Design review of the part built by this model. Coordinates are the model's own, in mm. Coordinates: 2 decimals unless noted, no trailing zeros. Write each loop counter-clockwise with the first axis right and the second up, starting at its lowest first coordinate (ties: lowest second). Pieces come first, ordered by that corner, then holes. Notation, with made-up numbers: (-20, -26.75) - (38, -26.75) arc R25 ccw to (38, -9.75) - close; hole circle Ø1 at (2, 9.5). An arc over 180 degrees is marked (long way). One line per item, written item: value.
from build123d import *

# Parameters (mm, degrees)
BOSS_EXTRUDE1_DEPTH                  = 166.33825
F_10_32_TAPPED_HOLE1_D               = 4.0386
F_10_32_TAPPED_HOLE1_DEPTH           = 16.34744
F_10_32_TAPPED_HOLE1_TIP             = 1.213317848
F_10_32_TAPPED_HOLE1_ON_FACE_2_D     = 4.0386
F_10_32_TAPPED_HOLE1_ON_FACE_2_DEPTH = 16.34744
F_10_32_TAPPED_HOLE1_ON_FACE_2_TIP   = 1.213317848
SKETCH5_W                            = 0.889
SKETCH5_H                            = 1.0033


with BuildPart() as part:
    # Sketch1 → Boss-Extrude1 (new, symmetric)
    with BuildSketch(Plane.XY):
        with BuildLine():
            ThreePointArc((0.93173274, 6.79441227), (0, 6.858), (-0.93173274, 6.79441227))
            Line((-0.93173274, 6.79441227), (-5.41826726, 4.204110358))
            ThreePointArc((-5.41826726, 4.204110358), (-5.939202219, 3.429), (-6.35, 2.590301913))
            Line((-6.35, 2.590301913), (-6.35, -2.590301913))
            ThreePointArc((-6.35, -2.590301913), (-5.939202219, -3.429), (-5.41826726, -4.204110358))
            Line((-5.41826726, -4.204110358), (-0.93173274, -6.79441227))
            ThreePointArc((-0.93173274, -6.79441227), (0, -6.858), (0.93173274, -6.79441227))
            Line((0.93173274, -6.79441227), (5.41826726, -4.204110358))
            ThreePointArc((5.41826726, -4.204110358), (5.939202219, -3.429), (6.35, -2.590301913))
            Line((6.35, -2.590301913), (6.35, 2.590301913))
            ThreePointArc((6.35, 2.590301913), (5.939202219, 3.429), (5.41826726, 4.204110358))
            Line((5.41826726, 4.204110358), (0.93173274, 6.79441227))
        make_face()
    extrude(amount=BOSS_EXTRUDE1_DEPTH, both=True)

    # #10-32 Tapped Hole1
    with Locations(Plane.XY.offset(166.33825)):
        with Locations((0, 0)):
            Hole(F_10_32_TAPPED_HOLE1_D / 2, depth=F_10_32_TAPPED_HOLE1_DEPTH)
            with Locations((0, 0, -(F_10_32_TAPPED_HOLE1_DEPTH + F_10_32_TAPPED_HOLE1_TIP / 2))):  # 118° drill point
                Cone(0, F_10_32_TAPPED_HOLE1_D / 2, F_10_32_TAPPED_HOLE1_TIP, mode=Mode.SUBTRACT)

    # #10-32 Tapped Hole1 on face 2
    with Locations(Plane(origin=(0, 0, -166.33825), x_dir=(-1, 0, 0), z_dir=(0, 0, -1))):
        with Locations((0, 0)):
            Hole(F_10_32_TAPPED_HOLE1_ON_FACE_2_D / 2, depth=F_10_32_TAPPED_HOLE1_ON_FACE_2_DEPTH)
            with Locations((0, 0, -(F_10_32_TAPPED_HOLE1_ON_FACE_2_DEPTH + F_10_32_TAPPED_HOLE1_ON_FACE_2_TIP / 2))):  # 118° drill point
                Cone(0, F_10_32_TAPPED_HOLE1_ON_FACE_2_D / 2, F_10_32_TAPPED_HOLE1_ON_FACE_2_TIP, mode=Mode.SUBTRACT)

    # Sketch5 → Cut-Revolve1 (revolve, cut)
    with BuildSketch(Plane(origin=(0, 0, 0), x_dir=(0, 0, -1), z_dir=(1, 0, 0)), mode=Mode.PRIVATE) as cut_revolve1_sk:
        with Locations((-164.30625, 6.35635)):
            Rectangle(SKETCH5_W, SKETCH5_H)
    revolve(cut_revolve1_sk.sketch.rotate(Axis((0, 0, 165.047176272), (0, 0, -1)), 90), axis=Axis((0, 0, 165.047176272), (0, 0, -1)), mode=Mode.SUBTRACT)


solid = part.part
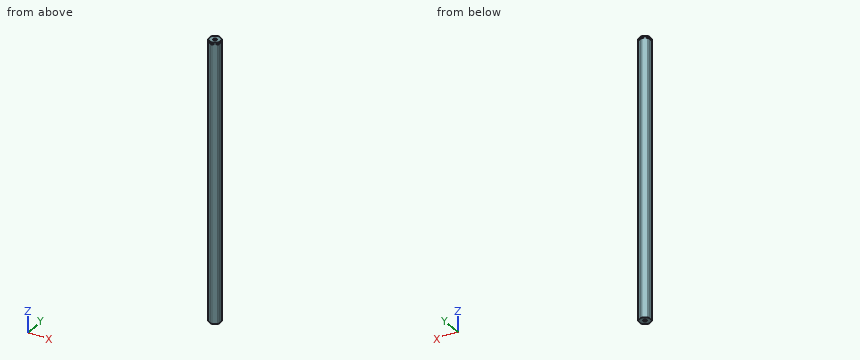
1. Insertion check: pin 1 Ø6 at (x, z) = (-4, -69) entering from +Y (3 decimals); pin 2 Ø3 at (x, z) = (-0.5, 48) entering from +Y. Each pin has a flat end and moves straight along its axis. Give the tip position at first contact, or say it passes through.
Answer block:
pin 1: stops at y = 6.755
pin 2: stops at y = 6.86
2. Wall thickness on line 1 along Y through (x, z) = (0, -162.5); line 2 along Z through (x, y) = (1.5, 6.25); line 3 along X through (y, z) = (0, 155): over which ranges is each line inside the solid? List them lowest first.
Answer block:
line 1: y = -6.86 to -2.02, 2.02 to 6.86
line 2: z = -166.34 to 163.86, 164.75 to 166.34
line 3: x = -6.35 to -2.02, 2.02 to 6.35
3. Consider section A-A, the plane z = 18.5. Write out the cut boundary in (x, y).
Answer block:
outline: (-6.35, -2.59) arc R6.86 ccw to (-5.42, -4.2) - (-0.93, -6.79) arc R6.86 ccw to (0.93, -6.79) - (5.42, -4.2) arc R6.86 ccw to (6.35, -2.59) - (6.35, 2.59) arc R6.86 ccw to (5.42, 4.2) - (0.93, 6.79) arc R6.86 ccw to (-0.93, 6.79) - (-5.42, 4.2) arc R6.86 ccw to (-6.35, 2.59) - close
